Here's how the part is built. I have some questions about the finished solid (model axes, mm). Face numbers are marked on the shaded views. Round coordinates to 2 decimals unless told otherwise and drop trailing zeros. Write each loop counter-clockwise with the first axis right and the second up, starting at its lowest first coordinate (ties: lowest second). Pieces come first, ordered by that corner, then holes. Notation, with made-up numbers: (42, 32) -> (50, 32) arc R31 ccw to (50, 70) -> close; hole circle Ø11 at (39.5, 12). An arc over 180 degrees is marked (long way). Answer in a Markdown table with one row per item.
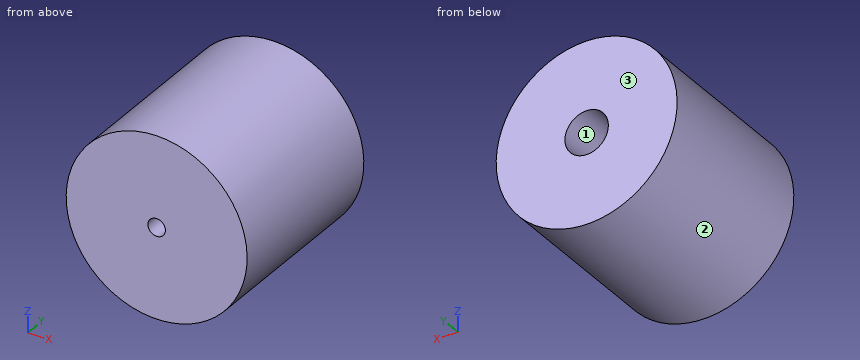
from build123d import *

# Parameters (mm, degrees)
SKETCH1_R           = 17.5
BOSS_EXTRUDE1_DEPTH = 35
SKETCH2_R           = 4.2
CUT_EXTRUDE1_DEPTH  = 10
SKETCH3_R           = 1.7
CUT_EXTRUDE2_DEPTH  = 26
CHAMFER1_SIZE       = 2.4892


with BuildPart() as part:
    # Sketch1 → Boss-Extrude1 (new body)
    with BuildSketch(Plane(origin=(0, 0, 0), x_dir=(1, 0, 0), z_dir=(0, 1, 0))):
        with Locations(Location((0, 0, 0), (0, 0, 270))):  # turned: the seam where the file's is
            Circle(SKETCH1_R)
    extrude(amount=BOSS_EXTRUDE1_DEPTH)

    # Sketch2 → Cut-Extrude1 (cut)
    with BuildSketch(Plane(origin=(0, 35, 0), x_dir=(1, 0, 0), z_dir=(0, 1, 0))):
        with Locations(Location((0, 0, 0), (0, 0, 270))):  # turned: the seam where the file's is
            Circle(SKETCH2_R)
    extrude(amount=-CUT_EXTRUDE1_DEPTH, mode=Mode.SUBTRACT)

    # Sketch3 → Cut-Extrude2 (cut, through all)
    with BuildSketch(Plane(origin=(0, 25, 0), x_dir=(1, 0, 0), z_dir=(0, 1, 0))):
        with Locations(Location((0, 0, 0), (0, 0, 270))):  # turned: the seam where the file's is
            Circle(SKETCH3_R)
    extrude(amount=-CUT_EXTRUDE2_DEPTH, mode=Mode.SUBTRACT)

    # Chamfer1
    chamfer1_edges = [part.edges().sort_by_distance(p)[0] for p in [
        (0, 25, -1.7),
    ]]
    chamfer(chamfer1_edges, length=CHAMFER1_SIZE)


solid = part.part
1) I want a section at D-D, the plane y = 7. List the corners of the cut face in (x, z) for me, and give its area (3 significant figures).
Response:
| item | result |
|---|---|
| outline | circle Ø35 at (0, 0); hole circle Ø3.4 at (0, 0) |
| area | 953 mm^2 |
2) We'd pull the mould along X, two halves only. Please class the marked faces 1, 2 and 3: +X half, -X half, draft (parallel to the pull), parting line (faces both ways), or undercut.
Response:
| item | result |
|---|---|
| face 1 | undercut |
| face 2 | parting line |
| face 3 | draft |
3) I want a section at C-C, the plane y = 31. List the corners of the cut face in (x, z) for me.
Response:
| item | result |
|---|---|
| outline | circle Ø35 at (0, 0); hole circle Ø8.4 at (0, 0) |
4) I need wall thicknesses on line 1 (X direction, y = 11, z = 0); line 2 (X direction, y = 28, z = 0); line 3 (Z direction, x = -0.5, y = 7). Which ranges of each line are inside material? Lowest first, please. Write a range as [from, to].
Response:
| item | result |
|---|---|
| line 1 | x = [-17.5, -1.7], [1.7, 17.5] |
| line 2 | x = [-17.5, -4.2], [4.2, 17.5] |
| line 3 | z = [-17.49, -1.62], [1.62, 17.49] |
5) For pin 1 (8 mm diameter, centred on x = -12.5, z = -13, fed in from +Y); pin 2 (4 mm diameter, centred on x = 0, z = 0, fed in from +Y); pin 3 (2 mm diameter, centred on x = -1.5, y = 4, fed in from +Z); pin 4 (3 mm diameter, centred on x = -13, y = 21, fed in from +Z), each with a flat end and sliding along its axis, tell me the tip position at first contact or that it passes through.
Response:
| item | result |
|---|---|
| pin 1 | stops at y = 35 |
| pin 2 | stops at y = 22.81 |
| pin 3 | stops at z = 17.49 |
| pin 4 | stops at z = 13.19 |
